from build123d import *

# Parameters (mm, degrees)
F2_DEPTH = 88.9
F3_R     = 40.697857
F4_DEPTH = 83.312


with BuildPart() as f2:
    # F1 (on face) → F2 (new body)
    with BuildSketch(Plane.XY):
        Polygon((25.532047, -40.773313), (44.621812, -17.978942), (46.667561, 11.682773), (30.887888, 36.882066), (3.310092, 47.993663), (-25.532047, 40.773313), (-44.621812, 17.978942), (-46.667561, -11.682773), (-30.887888, -36.882066), (-3.310092, -47.993663), align=None)
    extrude(amount=F2_DEPTH)

    # F3 (on face) → F4 (cut)
    with BuildSketch(Plane.XY.offset(88.9)):
        Circle(F3_R)
    extrude(amount=-F4_DEPTH, mode=Mode.SUBTRACT)


solid = f2.part
Source: CAD feature listing. Evaluate the final solid. Frame: model axes, mm. A direction names the side the tool comes from. Give positions to 0.01 mm unless a question says otherwise; leave off trailing zeros. Write each loop counter-clockwise with the first axis right and the second up, starting at its lowest first coordinate (ties: lowest second). Pieces come first, ordered by that corner, then holes. Notation, with made-up numbers: M 67.25,65 L 78.25,65 A20 ccw 78.25,78 Z; hole C 71,16 d10. An arc over 180 degrees is marked long. Return JSON: item names as keys, results as strings. Group by question number.
1) Set-up query: faces 1 (the face through (-8.82, -39.73, 47.83)), 2 (the face through (45.63, -3.36, 43.83)). Return all of +Z, -Z, +X, -X, +Y, -Y with unobstructed straight access to the full face (end or side cutting, diameter ignored); none if empty.
2) Draft query along X for faces 3 (the face through (-21, -35.3, 88.9)), 4 (the face through (17.29, 42.36, 43.83)), 5 (the face through (-1, 1, 5.588)), 6 (the face through (-10.909, 44.434, 43.828)). Return one class per face: released by +X, released by -X, zero draft, split by the parting line, or undercut.
3) Cut plane A-A, the plane z = 73.5. Output: boundary loops of the cut face in (x, y), then the cut area to 3 significant figures.
4) Cut plane C-C, the plane x = -19.5. Output: boundary loops of the cut face in (y, z), then the cut area to 3 significant figures.
5) Cut plane B-B, the plane y = 0. Output: boundary loops of the cut face in (x, z).
6) First-contact query: pin 1 Ø1.5 at (y, z) = (-31.5, 64.5) entering from +X; pin 2 Ø3 at (x, z) = (-20.5, 36.5) entering from -Y; pin 3 Ø12 at (y, z) = (-31.5, 25) entering from +X. Flat tips, straight axial feed; report the tip coordinate or a pass-through.
7) Ray query, L1, parallel to Z at x = 15, y = -37; L2, parallel to X at y = -23.5, z = 14.5; L3, parallel to Y at x = -7, z = 43.5. Return the intervals inside material, ascending.
Data:
{
 "1": {"face 1": "+Z", "face 2": "+Z, -Z, +X, -Y"},
 "2": {"face 3": "zero draft", "face 4": "released by +X", "face 5": "undercut", "face 6": "released by -X"},
 "3": {"outline": "M -46.67,-11.68 L -30.89,-36.88 L -3.31,-47.99 L 25.53,-40.77 L 44.62,-17.98 L 46.67,11.68 L 30.89,36.88 L 3.31,47.99 L -25.53,40.77 L -44.62,17.98 Z; hole C 0,0 d81.4", "area": "1,600 mm²"},
 "4": {"outline": "M -41.47,0 L 42.28,0 L 42.28,88.9 L 35.72,88.9 L 35.72,5.59 L -35.72,5.59 L -35.72,88.9 L -41.47,88.9 Z", "area": "1,490 mm²"},
 "5": {"outline": "M -45.86,0 L 45.86,0 L 45.86,88.9 L 40.7,88.9 L 40.7,5.59 L -40.7,5.59 L -40.7,88.9 L -45.86,88.9 Z"},
 "6": {"pin 1": "stops at x = 33.93", "pin 2": "stops at y = -41.67", "pin 3": "stops at x = 38.32"},
 "7": {"L1": "z = 0 to 5.59", "L2": "x = -39.27 to -33.23, 33.23 to 40", "L3": "y = -46.51 to -40.09, 40.09 to 45.41"}
}
